from build123d import *

# Parameters (mm, degrees)
SKETCH_1_R      = 4.5
SKETCH_1_R_2    = 4
EXTRUDE_1_DEPTH = 5


with BuildPart() as part:
    # 草图1 → 凸台-拉伸1 (new body)
    with BuildSketch(Plane(origin=(0, 0, 0), x_dir=(1, 0, 0), z_dir=(0, 1, 0))):
        with BuildLine():
            Line((-74, 10), (74, 10))
            ThreePointArc((74, 10), (84, 0), (74, -10))
            Line((74, -10), (-74, -10))
            ThreePointArc((-74, -10), (-84, 0), (-74, 10))
        make_face()
        with Locations(Location((74, 0, 0), (0, 0, 270))):
            Circle(SKETCH_1_R, mode=Mode.SUBTRACT)
        with Locations(Location((-74, 0, 0), (0, 0, 270))):
            Circle(SKETCH_1_R, mode=Mode.SUBTRACT)
        with Locations(Location((-24, 0, 0), (0, 0, 270))):
            Circle(SKETCH_1_R_2, mode=Mode.SUBTRACT)
        with Locations(Location((24, 0, 0), (0, 0, 90))):
            Circle(SKETCH_1_R_2, mode=Mode.SUBTRACT)
        with BuildLine():
            Line((-60, 5), (-36, 5))
            ThreePointArc((-36, 5), (-31, 0), (-36, -5))
            Line((-36, -5), (-60, -5))
            ThreePointArc((-60, -5), (-65, 0), (-60, 5))
        make_face(mode=Mode.SUBTRACT)
        with BuildLine():
            Line((-12, 5), (12, 5))
            ThreePointArc((12, 5), (17, 0), (12, -5))
            Line((12, -5), (-12, -5))
            ThreePointArc((-12, -5), (-17, 0), (-12, 5))
        make_face(mode=Mode.SUBTRACT)
        with BuildLine():
            Line((60, 5), (36, 5))
            ThreePointArc((36, 5), (31, 0), (36, -5))
            Line((36, -5), (60, -5))
            ThreePointArc((60, -5), (65, 0), (60, 5))
        make_face(mode=Mode.SUBTRACT)
    extrude(amount=EXTRUDE_1_DEPTH)


solid = part.part
Build history of the part. All positions in model axes, mm. A direction names the side the tool comes from. Give positions to 0.01 mm unless a question says otherwise; leave off trailing zeros. Order: outer loops, then holes, each group sorted by start corner. A loop starts at its lowest first (then second) coordinate and runs counter-clockwise, first axis right, second up. Notation, with made-up numbers: M 43.25,18 L 93.25,18 A13 cw 93.25,35 Z; hole C 55,8 d9. An arc over 180 degrees is marked long. Use one line per item in the form item = value.
Q1. Slice it at A-A, the plane x = 42. Write the cut outline in (y, z), and give its area (3 significant figures).
Conclusion:
outline = M 0,-10 L 5,-10 L 5,-5 L 0,-5 Z; M 0,5 L 5,5 L 5,10 L 0,10 Z
area = 50.0 mm2
Q2. Pull direction Z, two halves, no side cores. Call faces 1 (the flat face through (1, 2, 10)), 2 (the cylindrical face through (78.46, 2.46, -0.59)), 3 (the flat face through (-1, 2, -10)): released by +Z, released by -Z, zero draft, split by the parting line, or undercut.
Conclusion:
face_1 = released by +Z
face_2 = undercut
face_3 = released by -Z
Q3. Wall check: probe 1 along Z at (x, y) = (24, 1.45); probe 2 along Z at (x, y) = (59.5, 4.8); probe 3 along X at (y, z) = (3.2, 5.75). Give the ranges that are in metal, low to high.
Conclusion:
probe_1 = -10 to -4, 4 to 10
probe_2 = -10 to -5, 5 to 10
probe_3 = -82.18 to 82.18
Q4. Slice it at B-B, the plane y = 2.7. Write the cut outline in (x, z).
Conclusion:
outline = M -74,-10 L 74,-10 A10 ccw 74,10 L -74,10 A10 ccw Z; hole C -74,0 d9; hole M -60,-5 L -36,-5 A5 ccw -36,5 L -60,5 A5 ccw Z; hole C -24,0 d8; hole M -12,-5 L 12,-5 A5 ccw 12,5 L -12,5 A5 ccw Z; hole C 24,0 d8; hole M 36,-5 L 60,-5 A5 ccw 60,5 L 36,5 A5 ccw Z; hole C 74,0 d9
Q5. Which spindle directions (+Z, -Z, +X, -X, +Y, -Y) get a long thin tool onto all of the face, cutting with end or side? Do faces 4 (the cylindrical face through (84, 2, 0)), 5 (the flat face through (48, 2, -5)). Say none if no direction does.
Conclusion:
face_4 = +X, +Y, -Y
face_5 = +Y, -Y
Q6. Slice it at C-C, the plane z = 0.5. State how many separate pieces and enclosed holes the cut face has, and give its area (3 significant figures).
Conclusion:
separate_pieces = 8
enclosed_holes = 0
area = 162 mm2
Q7. Pin check, flat tip, straight feed: P1, Ø1, axis at x = -15.5, z = 1, coming from the -Y side. Stop position of the tip, or through.
Conclusion:
P1 = through
Q8. Slice it at D-D, the plane x = -24. Write the cut outline in (y, z).
Conclusion:
outline = M 0,-10 L 5,-10 L 5,-4 L 0,-4 Z; M 0,4 L 5,4 L 5,10 L 0,10 Z
